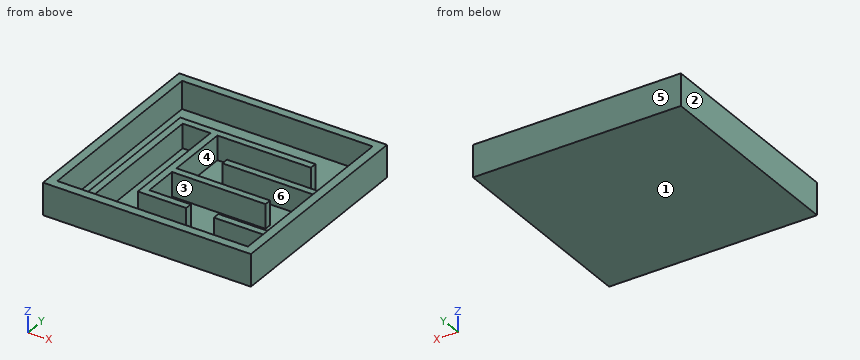
from build123d import *

# Parameters (mm, degrees)
F0_W     = 38.1
F0_H     = 38.1
F1_DEPTH = 0.79375
F2_W     = 38.1
F2_H     = 38.1
F2_W_2   = 34.925
F2_H_2   = 34.925
F3_DEPTH = 5.08
F4_W     = 17.145
F4_H     = 1.27
F4_W_2   = 9.5498631887
F5_DEPTH = 4.445
F4_R     = 1.27
F6_DEPTH = 0.396875


with BuildPart() as f1:
    # F0 (on Top) → F1 (new body)
    with BuildSketch(Plane.XY):
        with Locations((6.1000548303, -3.6594523599)):
            Rectangle(F0_W, F0_H)
    extrude(amount=F1_DEPTH)

    # F2 (on face) → F3 (join)
    with BuildSketch(Plane.XY.offset(0.79375)):
        with Locations((6.1000548303, -3.6594523599)):
            Rectangle(F2_W, F2_H)
        with Locations((6.1000548303, -3.6594523599)):
            Rectangle(F2_W_2, F2_H_2, mode=Mode.SUBTRACT)
    extrude(amount=F3_DEPTH)

    # F4 (on face) → F5 (join)
    with BuildSketch(Plane.XY.offset(0.79375)):
        Polygon((-6.2824451697, 5.5480476401), (-6.2824451697, -21.1219523599), (-5.0124451697, -21.1219523599), (-5.0124451697, 4.2780476401), (0.0675548303, 4.2780476401), (0.0675548303, -16.0419523599), (8.9326916416, -16.0419523599), (8.9326916416, -14.7719523599), (1.3375548303, -14.7719523599), (1.3375548303, -8.4219523599), (18.4825548303, -8.4219523599), (18.4825548303, -7.1519523599), (1.3375548303, -7.1519523599), (1.3375548303, 4.2780476401), (18.4825548303, 4.2780476401), (18.4825548303, 5.5480476401), (-5.0124451697, 5.5480476401), align=None)
        with Locations((14.9900548303, -1.4369523599)):
            Rectangle(F4_W, F4_H)
        with Locations((18.787623236, -15.4069523599)):
            Rectangle(F4_W_2, F4_H)
    extrude(amount=F5_DEPTH)

    # F4 (on face) → F6 (cut)
    with BuildSketch(Plane.XY.offset(0.79375)):
        with Locations((-8.8224451697, -17.4266919494)):
            Circle(F4_R)
        with Locations((-2.4724451697, 1.2010911014)):
            Circle(F4_R)
    extrude(amount=-F6_DEPTH, mode=Mode.SUBTRACT)


solid = f1.part
Here's how the part is built. I have some questions about the finished solid (model axes, mm). Face numbers are marked on the shaded views. A direction names the side the tool comes from. Coordinates: 2 decimals unless noted, no trailing zeros. Loops run counter-clockwise (first coordinate to the right, second up) from the corner with the lowest first, then second, coordinate; pieces in that order, holes last. Notation, with made-up numbers: (-34.5, -18) -> (-5.5, -18) arc R21 ccw to (-5.5, 20) -> close; hole circle Ø11 at (33.5, 32). An arc over 180 degrees is marked (long way). Use one line per item in the form item = value. Start each with the question number.
(1) We'd pull the mould along X, two halves only. Please class the marked faces 1, 2, 3 and 4: pulls with the +X half, pulls with the -X half, needs draft (parallel to the pull), parting line crosses it, or undercut.
(2) On a 3-axis mill with a long thin cutter (end or side, diameter ignored), from which of +Z, -Z, +X, -X, +Y, -Y can I reach the whole of each face in a straight line? I mean the marked faces 5 and 6. Say none if no direction works.
(3) If we section it at B-B (y = 9): Please give me the cut outline in (x, z), then the cut area to 3 significant figures.
(4) If we section it at C-C (x = 2): Please give me the cut outline in (y, z).
(5) If we section it at D-D (x = -5.5): Please give me the cut outline in (y, z).
(6) Please list where these lines run through material, in increasing order: line 1 along X through (y, z) = (-15, 1.9); line 2 along X through (y, z) = (2, 4.45); line 3 along Y through (x, z) = (4.5, 4.1).
(7) Will these pins go through, and if not, where does the flat tip stop? pin 1 (10 mm diameter, centred on x = 18, y = 6, fed in from +Z); pin 2 (1 mm diameter, centred on x = -8.5, y = -11, fed in from +Z).
Verdict:
q1.face_1 = needs draft
q1.face_2 = pulls with the -X half
q1.face_3 = undercut
q1.face_4 = undercut
q2.face_5 = +Z, -Z, +X, -X, +Y
q2.face_6 = +Z
q3.outline = (-12.95, 0) -> (25.15, 0) -> (25.15, 5.87) -> (23.56, 5.87) -> (23.56, 0.79) -> (-11.36, 0.79) -> (-11.36, 5.87) -> (-12.95, 5.87) -> close
q3.area = 46.4 mm²
q4.outline = (-22.71, 0) -> (15.39, 0) -> (15.39, 5.87) -> (13.8, 5.87) -> (13.8, 0.79) -> (5.55, 0.79) -> (5.55, 5.24) -> (4.28, 5.24) -> (4.28, 0.79) -> (-7.15, 0.79) -> (-7.15, 5.24) -> (-8.42, 5.24) -> (-8.42, 0.79) -> (-14.77, 0.79) -> (-14.77, 5.24) -> (-16.04, 5.24) -> (-16.04, 0.79) -> (-21.12, 0.79) -> (-21.12, 5.87) -> (-22.71, 5.87) -> close
q5.outline = (-22.71, 0) -> (15.39, 0) -> (15.39, 5.87) -> (13.8, 5.87) -> (13.8, 0.79) -> (5.55, 0.79) -> (5.55, 5.24) -> (-21.12, 5.24) -> (-21.12, 5.87) -> (-22.71, 5.87) -> close
q6.line_1 = -12.95 to -11.36, -6.28 to -5.01, 0.07 to 8.93, 14.01 to 25.15
q6.line_2 = -12.95 to -11.36, -6.28 to -5.01, 0.07 to 1.34, 23.56 to 25.15
q6.line_3 = -22.71 to -21.12, -16.04 to -14.77, -8.42 to -7.15, 4.28 to 5.55, 13.8 to 15.39
q7.pin_1 = 5.24
q7.pin_2 = 0.79
